from build123d import *

# Parameters (mm, degrees)
SKETCH1_W                       = 20
SKETCH1_H                       = 20
BOSS_EXTRUDE1_DEPTH             = 20
CUT_EXTRUDE1_DEPTH              = 43.426406871
CUT_EXTRUDE1_DEPTH_BACK         = 43.426406871
CUT_EXTRUDE3_DEPTH              = 25.494897428
CUT_EXTRUDE3_DEPTH_BACK         = 25.494897428
SKETCH3_W                       = 15
SKETCH3_H                       = 15.1
BOSS_EXTRUDE3_DEPTH             = 6.9
BOSS_EXTRUDE3_DEPTH_BACK        = 6.9
SKETCH5_R                       = 2.38
FILLET1_R                       = 0.5
SKETCH7_W                       = 9.8
SKETCH7_H                       = 10
BOSS_EXTRUDE4_DEPTH             = 30
BOSS_EXTRUDE5_REACH             = 42.898
BOSS_EXTRUDE5_DIRECTION_2_REACH = 42.898
CUT_EXTRUDE4_DEPTH              = 43.621708084
CUT_EXTRUDE4_DEPTH_BACK         = 43.621708084
FILLET2_R                       = 3


with BuildPart() as part:
    # Sketch1 → Boss-Extrude1 (new, symmetric)
    with BuildSketch(Plane.XY):
        Rectangle(SKETCH1_W, SKETCH1_H)
    extrude(amount=BOSS_EXTRUDE1_DEPTH, both=True)

    # Sketch2 → Cut-Extrude1 (cut, two sides: drawn at the far end of the back side and taken through both)
    with BuildSketch(Plane.XY.offset(20).offset(-CUT_EXTRUDE1_DEPTH_BACK)):
        with BuildLine():
            ThreePointArc((0, -5), (-5, 0), (0, 5))
            Line((0, 5), (10, 5))
            Line((10, 5), (10, 10))
            Line((10, 10), (-10, 10))
            Line((-10, 10), (-10, -10))
            Line((-10, -10), (10, -10))
            Line((10, -10), (10, -5))
            Line((10, -5), (0, -5))
        make_face()
    extrude(amount=CUT_EXTRUDE1_DEPTH + CUT_EXTRUDE1_DEPTH_BACK, mode=Mode.SUBTRACT)

    # Sketch3 → Cut-Extrude3 (cut, two sides: drawn at the far end of the back side and taken through both)
    with BuildSketch(Plane(origin=(0, 5, 0), x_dir=(1, 0, 0), z_dir=(0, 1, 0)).offset(-CUT_EXTRUDE3_DEPTH_BACK)):
        with Locations((2.5, 12.45)):
            Rectangle(SKETCH3_W, SKETCH3_H)
        with Locations((2.5, -12.45)):
            Rectangle(SKETCH3_W, SKETCH3_H)
    extrude(amount=CUT_EXTRUDE3_DEPTH + CUT_EXTRUDE3_DEPTH_BACK, mode=Mode.SUBTRACT)

    # Sketch5 → Boss-Extrude3 (add, two sides: drawn at the far end of the back side and taken through both)
    with BuildSketch(Plane.XY.offset(-BOSS_EXTRUDE3_DEPTH_BACK)):
        Circle(SKETCH5_R)
    extrude(amount=BOSS_EXTRUDE3_DEPTH + BOSS_EXTRUDE3_DEPTH_BACK)

    # Fillet1
    fillet1_edges = [part.edges().sort_by_distance(p)[0] for p in [
        (-2.38, 0, 6.9),
        (-2.38, 0, -6.9),
    ]]
    fillet(fillet1_edges, radius=FILLET1_R)

    # Sketch7 → Boss-Extrude4 (add)
    with BuildSketch(Plane(origin=(10, 0, 0), x_dir=(0, 0, -1), z_dir=(1, 0, 0))):
        Rectangle(SKETCH7_W, SKETCH7_H)
    extrude(amount=BOSS_EXTRUDE4_DEPTH)

    # Boss-Extrude5: up to this face of the body (flat: up to its plane)
    boss_extrude5_end = Plane(part.part.faces().sort_by_distance((18.783256068, 0, 4.9))[0])
    # Sketch11 → Boss-Extrude5 (add, up to the picked face)
    with BuildSketch(Plane.XY, mode=Mode.PRIVATE) as boss_extrude5_sk1:
        with BuildLine():
            Line((40, 9), (40, -9))
            ThreePointArc((40, -9), (36, -13), (32, -9))
            Line((32, -9), (32, 9))
            ThreePointArc((32, 9), (36, 13), (40, 9))
        make_face()
    boss_extrude5_tool1 = split(extrude(boss_extrude5_sk1.sketch, amount=BOSS_EXTRUDE5_REACH, mode=Mode.PRIVATE), bisect_by=boss_extrude5_end, keep=Keep.BOTH, mode=Mode.PRIVATE)
    add(boss_extrude5_tool1.solids().sort_by(Axis((36, 0, 0), (0, 0, 1)))[0])

    # Boss-Extrude5 direction 2: up to this face of the body (flat: up to its plane)
    boss_extrude5_direction_2_end = Plane(part.part.faces().sort_by_distance((18.783256068, 0, -4.9))[0])
    # Sketch11 → Boss-Extrude5 direction 2 (add, up to the picked face)
    with BuildSketch(Plane.XY, mode=Mode.PRIVATE) as boss_extrude5_direction_2_sk1:
        with BuildLine():
            Line((40, 9), (40, -9))
            ThreePointArc((40, -9), (36, -13), (32, -9))
            Line((32, -9), (32, 9))
            ThreePointArc((32, 9), (36, 13), (40, 9))
        make_face()
    boss_extrude5_direction_2_tool1 = split(extrude(boss_extrude5_direction_2_sk1.sketch, amount=-BOSS_EXTRUDE5_DIRECTION_2_REACH, mode=Mode.PRIVATE), bisect_by=boss_extrude5_direction_2_end, keep=Keep.BOTH, mode=Mode.PRIVATE)
    add(boss_extrude5_direction_2_tool1.solids().sort_by(Axis((36, 0, 0), (0, 0, -1)))[0])

    # Sketch13 → Cut-Extrude4 (cut, two sides: drawn at the far end of the back side and taken through both)
    with BuildSketch(Plane.XY.offset(-CUT_EXTRUDE4_DEPTH_BACK)):
        with BuildLine():
            ThreePointArc((37.5, 6.95), (37.060660172, 8.010660172), (36, 8.45))
            Line((36, 8.45), (36, 5.45))
            ThreePointArc((36, 5.45), (37.060660172, 5.889339828), (37.5, 6.95))
        make_face()
        with BuildLine():
            Line((36, 5.45), (36, 8.45))
            ThreePointArc((36, 8.45), (34.5, 6.95), (36, 5.45))
        make_face()
        with BuildLine():
            ThreePointArc((37.5, -6.95), (37.060660172, -5.889339828), (36, -5.45))
            Line((36, -5.45), (36, -8.45))
            ThreePointArc((36, -8.45), (37.060660172, -8.010660172), (37.5, -6.95))
        make_face()
        with BuildLine():
            Line((36, -8.45), (36, -5.45))
            ThreePointArc((36, -5.45), (34.5, -6.95), (36, -8.45))
        make_face()
    extrude(amount=CUT_EXTRUDE4_DEPTH + CUT_EXTRUDE4_DEPTH_BACK, mode=Mode.SUBTRACT)

    # Fillet2
    fillet2_edges = [part.edges().sort_by_distance(p)[0] for p in [
        (32, -5, 0),
        (32, 5, 0),
    ]]
    fillet(fillet2_edges, radius=FILLET2_R)


solid = part.part
Model file for the job. Use its own axes, mm. A direction names the side the tool comes from. Round coordinates to 2 decimals unless told otherwise and drop trailing zeros. Loops run counter-clockwise (first coordinate to the right, second up) from the corner with the lowest first, then second, coordinate; pieces in that order, holes last.
1. Tool access for faces 1 (the flat face through (32, -8.5, -0.1)), 2 (the cylindrical face through (-0.516, -2.323, 5.64)), 3 (the flat face through (32, 8.5, 0.1)): list every direction of +Z, -Z, +X, -X, +Y, -Y with a clear straight run to the whole face (end or side of a thin tool).
Check values:
face 1: +Z, -Z, -X, -Y
face 2: +Z
face 3: +Z, -Z, -X, +Y
2. Band-saw the part on B-B, the plane x = 36.5. List the corners of the cut face in (y, z).
Check values:
outline: (-12.97, -4.9) - (-8.36, -4.9) - (-8.36, 4.9) - (-12.97, 4.9) - close; (-5.54, -4.9) - (5.54, -4.9) - (5.54, 4.9) - (-5.54, 4.9) - close; (8.36, -4.9) - (12.97, -4.9) - (12.97, 4.9) - (8.36, 4.9) - close
3. Band-saw the part on A-A, the plane y = 0. List the corners of the cut face in (x, z), and give its area (3 significant figures).
Check values:
outline: (-5, -4.9) - (-2.38, -4.9) - (-2.38, -6.4) arc R0.5 ccw to (-1.88, -6.9) - (1.88, -6.9) arc R0.5 ccw to (2.38, -6.4) - (2.38, -4.9) - (40, -4.9) - (40, 4.9) - (2.38, 4.9) - (2.38, 6.4) arc R0.5 ccw to (1.88, 6.9) - (-1.88, 6.9) arc R0.5 ccw to (-2.38, 6.4) - (-2.38, 4.9) - (-5, 4.9) - close
area: 460 mm2
4. Drop flat-ended pins along their axis: P1, Ø5, axis at y = 6.5, z = -5, coming from the -X side; P2, Ø8, axis at x = 25.5, y = -5, coming from the -Z side; P3, Ø5, axis at x = 20.5, z = -2.5, coming from the +Y side. Give the stop position or say it passes through.
Check values:
P1: stops at x = -3
P2: stops at z = -4.9
P3: stops at y = 5
5. Band-saw the part on C-C, the plane x = 9. List the corners of the cut face in (y, z), and give its area (3 significant figures).
Check values:
outline: (-5, -4.9) - (5, -4.9) - (5, 4.9) - (-5, 4.9) - close
area: 98.0 mm2
6. Wall check: probe 1 along Z at (x, y) = (2.5, 0.5); probe 2 along X at (y, z) = (5.75, -3.5); probe 3 along Y at (x, z) = (16.5, -2.25). Give the ranges that are in metal, low to high.
Check values:
probe 1: z = -4.9 to 4.9
probe 2: x = 30.98 to 35.1, 36.9 to 40
probe 3: y = -5 to 5
7. Band-saw the part on D-D, the plane z = 5.75. List the corners of the cut face in (x, y).
Check values:
outline: circle Ø4.76 at (0, 0)
